Work out the finished part from the listing and answer in its coordinate system (mm). A direction names the side the tool comes from. Round coordinates to 2 decimals unless told otherwise and drop trailing zeros. Order: outer loops, then holes, each group sorted by start corner. A loop starts at its lowest first (then second) coordinate and runs counter-clockwise, first axis right, second up. Notation, with made-up numbers: M -21,37.5 L 21,37.5 A11 cw 21,55.5 Z; hole C -28.5,-0.5 d3. An arc over 180 degrees is marked long. Return JSON: item names as keys, results as strings.
from build123d import *

# Parameters (mm, degrees)
SKETCH_1_W           = 220
SKETCH_1_H           = 70
EXTRUDE_1_DEPTH      = 3
EXTRUDE_2_DEPTH      = 25
EXTRUDE_2_DEPTH_BACK = 25
SKETCH_6_W           = 30
SKETCH_6_H           = 37.527767497
CUT_EXTRUDE_4_DEPTH  = 221
SKETCH_7_R           = 35
CUT_EXTRUDE_5_DEPTH  = 4
SKETCH_8_W           = 3
SKETCH_8_H           = 40
EXTRUDE_3_DEPTH      = 65
SKETCH_9_R           = 1.5
CUT_EXTRUDE_6_DEPTH  = 4
FILLET_5_R           = 1
SKETCH_10_W          = 65
SKETCH_10_H          = 20
CUT_EXTRUDE_7_DEPTH  = 4
SKETCH_11_W          = 132.48262102
SKETCH_11_H          = 20
CUT_EXTRUDE_8_DEPTH  = 25
SKETCH_12_W          = 48
SKETCH_12_H          = 37
CUT_EXTRUDE_9_DEPTH  = 30


with BuildPart() as part:
    # 草图1 → 凸台-拉伸1 (new body)
    with BuildSketch(Plane(origin=(0, 0, 0), x_dir=(1, 0, 0), z_dir=(0, 1, 0))):
        with Locations((27.295373665, 0)):
            Rectangle(SKETCH_1_W, SKETCH_1_H)
    extrude(amount=EXTRUDE_1_DEPTH)

    # 草图2 → 凸台-拉伸2 (add, two sides)
    with BuildSketch(Plane.XY) as extrude_2_sk:
        Polygon((-82.704626335, 40.527767497), (-82.704626335, 3), (-17.704626335, 3), align=None)
    extrude(amount=EXTRUDE_2_DEPTH)
    extrude(extrude_2_sk.sketch, amount=-EXTRUDE_2_DEPTH_BACK)

    # 草图6 → 切除-拉伸4 (cut, through all)
    with BuildSketch(Plane.ZY.offset(82.704626335)):
        with Locations((0, 21.763883748)):
            Rectangle(SKETCH_6_W, SKETCH_6_H)
    extrude(amount=-CUT_EXTRUDE_4_DEPTH, mode=Mode.SUBTRACT)

    # 草图7 → 切除-拉伸5 (cut, through all)
    with BuildSketch(Plane(origin=(0, 3, 0), x_dir=(1, 0, 0), z_dir=(0, 1, 0))):
        with Locations((25.295373665, 51)):
            Circle(SKETCH_7_R)
        with Locations((25.295373665, -51)):
            Circle(SKETCH_7_R)
    extrude(amount=-CUT_EXTRUDE_5_DEPTH, mode=Mode.SUBTRACT)

    # 草图8 → 凸台-拉伸3 (add)
    with BuildSketch(Plane.ZY.offset(82.704626335)):
        with Locations((36.5, 20)):
            Rectangle(SKETCH_8_W, SKETCH_8_H)
        with Locations((-36.5, 20)):
            Rectangle(SKETCH_8_W, SKETCH_8_H)
    extrude(amount=-EXTRUDE_3_DEPTH)

    # 草图9 → 切除-拉伸6 (cut, through all)
    with BuildSketch(Plane(origin=(0, 3, 0), x_dir=(1, 0, 0), z_dir=(0, 1, 0))):
        with Locations((-74.766784803, 29.860059225)):
            Circle(SKETCH_9_R)
        with Locations((-54.766784803, 29.860059225)):
            Circle(SKETCH_9_R)
        with Locations((-34.766784803, 29.860059225)):
            Circle(SKETCH_9_R)
        with Locations((-34.766784803, -29.860059225)):
            Circle(SKETCH_9_R)
        with Locations((-54.766784803, -29.860059225)):
            Circle(SKETCH_9_R)
        with Locations((-74.766784803, -29.860059225)):
            Circle(SKETCH_9_R)
        with Locations((68.031562246, 22)):
            Circle(SKETCH_9_R)
        with Locations((88.031562246, 22)):
            Circle(SKETCH_9_R)
        with Locations((108.031562246, 22)):
            Circle(SKETCH_9_R)
        with Locations((108.031562246, -22)):
            Circle(SKETCH_9_R)
        with Locations((88.031562246, -22)):
            Circle(SKETCH_9_R)
        with Locations((68.031562246, -22)):
            Circle(SKETCH_9_R)
        with Locations((128.031562246, 22)):
            Circle(SKETCH_9_R)
        with Locations((128.031562246, -22)):
            Circle(SKETCH_9_R)
    extrude(amount=-CUT_EXTRUDE_6_DEPTH, mode=Mode.SUBTRACT)

    # 圆角5
    fillet_5_edges = [part.edges().sort_by_distance(p)[0] for p in [
        (-50.204626335, 21.763883749, -25),
        (-50.204626335, 21.763883749, 25),
        (-50.204626335, 21.763883749, -15),
        (-50.204626335, 21.763883749, 15),
    ]]
    fillet(fillet_5_edges, radius=FILLET_5_R)

    # 草图10 → 切除-拉伸7 (cut, through all)
    with BuildSketch(Plane(origin=(0, 3, 0), x_dir=(1, 0, 0), z_dir=(0, 1, 0))):
        with Locations((-50.204626335, 0)):
            Rectangle(SKETCH_10_W, SKETCH_10_H)
    extrude(amount=-CUT_EXTRUDE_7_DEPTH, mode=Mode.SUBTRACT)

    # 草图11 → 切除-拉伸8 (cut)
    with BuildSketch(Plane(origin=(0, 0, 0), x_dir=(1, 0, 0), z_dir=(0, 1, 0))):
        with Locations((48.536684175, 0)):
            Rectangle(SKETCH_11_W, SKETCH_11_H)
    extrude(amount=CUT_EXTRUDE_8_DEPTH, mode=Mode.SUBTRACT)

    # 草图12 → 切除-拉伸9 (cut)
    with BuildSketch(Plane(origin=(0, 0, 0), x_dir=(1, 0, 0), z_dir=(0, 1, 0))):
        with Locations((80.777994685, -0.5)):
            Rectangle(SKETCH_12_W, SKETCH_12_H)
    extrude(amount=CUT_EXTRUDE_9_DEPTH, mode=Mode.SUBTRACT)


solid = part.part
Item 1: Find section D-D (x = 12.5). Determine the outline of the cut face in (y, z).
Output:
{"outline": "M 0,-18.42 L 3,-18.42 L 3,-10 L 0,-10 Z; M 0,10 L 3,10 L 3,18.42 L 0,18.42 Z"}
Item 2: Each of these flat-tipped pins is pushed along its axis until it touches: pin 1 (3 mm diameter, centred on y = 14.5, z = -25, fed in from +X); pin 2 (3.5 mm diameter, centred on x = 71.5, y = 1.5, fed in from -Z); pin 3 (12 mm diameter, centred on x = 26.5, z = 11.5, fed in from +Y). Where does it stop, or does it pass through?
Output:
{"pin 1": "stops at x = -35.41", "pin 2": "stops at z = -35", "pin 3": "stops at y = 3"}
Item 3: Find section A-A (x = 97). Determine the outline of the cut face in (y, z).
Output:
{"outline": "M 0,-35 L 3,-35 L 3,-18 L 0,-18 Z; M 0,19 L 3,19 L 3,35 L 0,35 Z"}
Item 4: Which of the six approach directions +Z, -Z, +X, -X, +Y, -Y give full straight-line access (tool end or side, diameter ignored) to faces 5 (the flat face through (-49.75, 21.5, 20.06)), 6 (the flat face through (-66, 13, -25)), 7 (the flat face through (-82.705, 21, 24))?
Output:
{"face 5": "+X, +Y", "face 6": "+X, -X, +Y", "face 7": "+Z, -Z, -X, +Y, -Y"}
Item 5: Consider line 1 along X through (y, z) = (2.1, -22); line 2 along Z through (x, y) = (-46.5, 31.5); line 3 along Y through (x, z) = (76, -30.5). Determine where each line is inside the solid, lowest interval first. Write a range as [from, to].
Output:
{"line 1": "x = [-82.7, 5.7], [44.89, 66.53], [69.53, 86.53], [89.53, 106.53], [109.53, 126.53], [129.53, 137.3]", "line 2": "z = [-38, -35], [35, 38]", "line 3": "y = [0, 3]"}
Item 6: The mould has two halves that part along Z. Classify faces 1 (the flat face through (-59, 17, 15)), 2 (the flat face through (-51, 20, -38)), 3 (the flat face through (50, 0, 16)), 4 (the cylindrical face through (-50.81, 21.77, 24.71)): pulls with the +Z half, pulls with the -Z half, needs draft (parallel to the pull), parting line crosses it, or undercut.
Output:
{"face 1": "undercut", "face 2": "pulls with the -Z half", "face 3": "needs draft", "face 4": "undercut"}
Item 7: Find section B-B (z = 5). Determine the outline of the cut face in (x, y), plus the area to 3 significant figures.
Output:
{"outline": "M 114.78,0 L 137.3,0 L 137.3,3 L 114.78,3 Z", "area": "67.6 mm^2"}
Item 8: Find section C-C (y = 35). State how many separate pieces and enclosed holes the cut face has, plus the area to 3 significant figures.
Output:
{"separate pieces": "4", "enclosed holes": "0", "area": "580 mm^2"}
